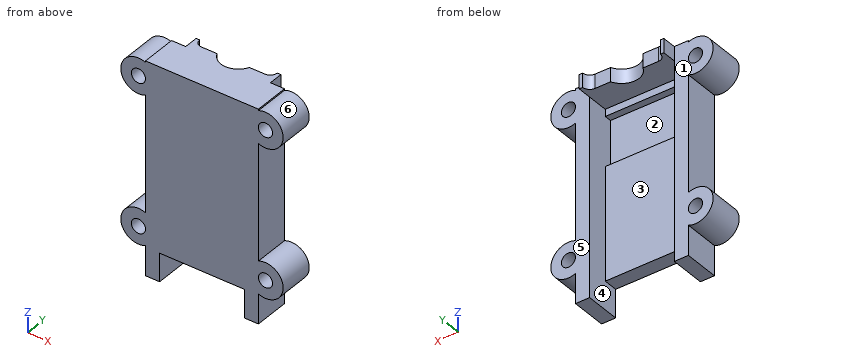
Autodesk Inventor part; units mm, degrees
ref_plane "YZ Plane" through (0, 0, 0) normal (1, 0, 0) x (0, 1, 0)
ref_plane "XZ Plane" through (0, 0, 0) normal (0, 1, 0) x (-1, 0, 0)
ref_plane "XY Plane" through (0, 0, 0) normal (0, 0, 1) x (1, 0, 0)
sketch "Sketch1" plane through (0, 0, 0) normal (0, 1, 0) x (-1, 0, 0)
  line L0 (8, 15) -> (-8, 15)
  line L1 (-8, 15) -> (-8, -15)
  line L2 (-8, -15) -> (8, -15)
  line L3 (8, -15) -> (8, 15)
  line L4 (8, 15) -> (-8, -15) construction
  line L5 (-8, 15) -> (8, -15) construction
  point P0 (0, 0)
  dimension "d0" = 16
  dimension "d1" = 30
extrude "Extrusion1" add sketch "Sketch1" along normal blind 2
sketch "Sketch2" plane through (0, 2, 0) normal (0, 1, 0) x (1, 0, 0)
  line L0 (8, 15) -> (-8, 15)
  line L1 (-6, 15) -> (6, 15)
  line L2 (6, 15) -> (6, -13)
  line L3 (6, -13) -> (-6, -13)
  line L4 (-6, -13) -> (-6, 15)
  line L5 (8, -15) -> (8, 15)
  line L6 (-8, 15) -> (-8, -15)
  line L7 (-8, -15) -> (8, -15)
  point P0 (0, 0)
  dimension "d4" = 2
  dimension "d5" = 2
  dimension "d6" = 2
extrude "Extrusion2" add sketch "Sketch2" along normal blind 3 contours L5 L7 L6 L0 L4 L3 L2
sketch "Sketch4" plane through (0, 5, 0) normal (0, 1, 0) x (1, 0, 0)
  line L0 (6, -13) -> (-6, -13)
  line L1 (-8, -15) -> (8, -15)
  line L2 (-6, -13) -> (6, -13)
  line L3 (6, -13) -> (6, -15)
  line L4 (6, -15) -> (-6, -15)
  line L5 (-6, -15) -> (-6, -13)
  line L6 (6, 15) -> (6, -13)
  point P0 (0, 0)
extrude "Extrusion3" add sketch "Sketch4" along normal blind 2
sketch "Sketch3" plane through (-8, 0, 15) normal (0, 0, 1) x (1, 0, 0)
  line L0 (14, 2) -> (2, 2) construction
  line L1 (2, 2) -> (14, 2) construction
  circle A0 centre (8, 7) radius 2.5
  line L2 (8, 11.4) -> (8, -1.9) construction
  line L3 (3.5, 7) -> (12.5, 7) construction
  circle A1 centre (3.5, 7) radius 1
  circle A2 centre (12.5, 7) radius 1
  line L4 (3.5, 8) -> (5.7087, 8)
  line L5 (12.5, 8) -> (10.2913, 8)
  line L6 (12.5, 6) -> (10.2913, 6)
  line L7 (5.7087, 6) -> (3.5, 6)
  point P0 (8, 0)
  dimension "d9" = 5
  dimension "d10" = 5
  dimension "d11" = 9
  dimension "d12" = 2
  dimension "d13" = 2
extrude "Extrusion4" cut sketch "Sketch3" against normal up to next
sketch "Sketch8" plane through (0, 2, 0) normal (0, 1, 0) x (1, 0, 0)
  line L0 (-6, 15) -> (-6, -13)
  line L1 (6, -13) -> (6, 15)
  line L2 (-6, 15) -> (6, 15)
  line L3 (6, 15) -> (6, 11)
  line L4 (6, 11) -> (-6, 11)
  line L5 (-6, 11) -> (-6, 15)
  line L6 (-2.2913, -13) -> (2.2913, -13)
  point P0 (0, 0)
  dimension "d28" = 24
extrude "Extrusion7" cut sketch "Sketch8" against normal up to next
sketch "Sketch9" plane through (0, 2, 0) normal (0, 1, 0) x (1, 0, 0)
  line L0 (-6, 11) -> (-6, -13)
  line L1 (6, -13) -> (6, 11)
  line L2 (-6, -12) -> (6, -12)
  line L3 (6, -12) -> (6, -5)
  line L4 (6, -5) -> (-6, -5)
  line L5 (-6, -5) -> (-6, -12)
  line L6 (-2.2913, -13) -> (2.2913, -13)
  point P0 (0, 0)
  point P1 (-6, -5)
  dimension "d31" = 1
  dimension "d32" = 7
extrude "Extrusion8" cut sketch "Sketch9" against normal blind 1
sketch "Sketch10" plane through (0, 0, 0) normal (0, -1, 0) x (1, 0, 0)
  circle A0 centre (-9, 12.5) radius 1
  circle A1 centre (-9, 12.5) radius 2.5
  line L0 (-8, -15) -> (-8, 15)
  line L1 (-8, 15) -> (8, 15)
  line L2 (8, 15) -> (8, -15)
  line L3 (-8, 15) -> (-6, 15)
  circle A2 centre (-9, -8.5) radius 1
  circle A3 centre (-9, -8.5) radius 2.5
  circle A4 centre (9, 12.5) radius 1
  circle A5 centre (9, 12.5) radius 2.5
  circle A6 centre (9, -8.5) radius 1
  circle A7 centre (9, -8.5) radius 2.5
  line L4 (6, -11) -> (-6, -11)
  point P0 (0, 0)
  point P1 (-8, -6)
  point P2 (10, 15)
  point P3 (10, -6)
  point P4 (-8, 12.5)
  point P5 (-8, 14.7913)
  point P6 (-8, 10.2087)
  point P7 (-8, -6.2087)
  point P8 (-8, -10.7913)
  point P9 (-8, -8.5)
  point P10 (8, 14.7913)
  point P11 (8, 12.5)
  point P12 (8, 10.2087)
  dimension "d35" = 2
  dimension "d36" = 1.5
  dimension "d38" = 16
  dimension "d41" = 21
  dimension "d44" = 18
  dimension "d49" = 26
extrude "Extrusion9" add sketch "Sketch10" against normal up to surface (5 mm away) contours L0 A1 | A7 L2 | L2 A7 | A5 L2 | L0 A3 picked at (-10.9649, 12.2158) picked at (10.9649, 12.2158) picked at (-10.9649, -8.7842)
equation "\"d5\" = d4"
equation "\"d6\" = d4"
equation "\"d41\" = -2 * d36 + d49 - d35"
properties part number "motor_top"
The model under review builds one solid part; all positions refer to its coordinate system, in mm. Face numbers are marked on the shaded views. A direction names the side the tool comes from. Give positions to 0.01 mm unless a question says otherwise; leave off trailing zeros. Write each loop counter-clockwise with the first axis right and the second up, starting at its lowest first coordinate (ties: lowest second). Pieces come first, ordered by that corner, then holes.
(1) Consider section D-D, the plane z = 12.5. Give the boundary of the cut face in (x, y), and give its area (3 significant figures).
(2) Tool access review of the marked faces 1, 2 and 3: name each direction out of +Z, -Z, +X, -X, +Y, -Y from which nothing blocks a thin tool from reaching the whole face with its end or side.
(3) To check wall thickness, follow L1, parallel to Z at x = -9, y = 2.6; L2, parallel to Z at x = 8.25, y = 0.5; L3, parallel to X at y = 3.5, z = -8. State the ranges of each line that lie inside material, in increasing order.
(4) The part is to be moulded in two halves that separate along X. For the marked faces 4, 5 and 6, say which applies: released by +X, released by -X, zero draft, split by the parting line, or undercut.
(5) For P1, Ø0.6, axis at x = 3.5, z = 14, coming from the +Y side; P2, Ø1, axis at x = 1, y = 1, coming from the -Z side; P3, Ø1.5, axis at x = 3.5, z = -3, coming from the +Y side; P4, Ø1.6, axis at x = 10, z = 6, coming from the +Y side, all flat-tipped, find the tip position at first contact; note any pin that passes through.
(6) Consider section A-A, the plane x = -9. Give the boundary of the cut face in (y, z).
(7) Consider section B-B, the plane z = 9.25. Give the boundary of the cut face in (x, y).
(8) Consider section C-C, the plane y = 3.75. Give the boundary of the cut face in (x, z).
Returned:
1. outline: (-11.5, 0) - (-10, 0) - (-10, 5) - (-11.5, 5) - close; (-8, 0) - (8, 0) - (8, 5) - (6, 5) - (6, 2) - (-6, 2) - (-6, 5) - (-8, 5) - close; (10, 0) - (11.5, 0) - (11.5, 5) - (10, 5) - close
1. area: 59.0 mm2
2. face 1: +Z, -Z, -X, +Y
2. face 2: +Y
2. face 3: -Z, +Y
3. L1: z = -11 to -9.5, -7.5 to -6, 10 to 11.5, 13.5 to 15
3. L2: z = -10.88 to -9.16, -7.84 to -6.12, 10.12 to 11.84, 13.16 to 14.88
3. L3: x = -11.45 to -9.87, -8.13 to -6, 6 to 8.13, 9.87 to 11.45
4. face 4: undercut
4. face 5: zero draft
4. face 6: undercut
5. P1: stops at y = 6
5. P2: stops at z = -11
5. P3: stops at y = 2
5. P4: passes through
6. outline: (0, -11) - (5, -11) - (5, -9.5) - (0, -9.5) - close; (0, -7.5) - (5, -7.5) - (5, -6) - (0, -6) - close; (0, 10) - (5, 10) - (5, 11.5) - (0, 11.5) - close; (0, 13.5) - (5, 13.5) - (5, 15) - (0, 15) - close
7. outline: (-8, 0) - (8, 0) - (8, 5) - (6, 5) - (6, 1) - (-6, 1) - (-6, 5) - (-8, 5) - close
8. outline: (-8, -15) - (-6, -15) - (-6, 13) - (6, 13) - (6, -15) - (8, -15) - (8, -10.79) arc R2.5 ccw (long way) to (8, -6.21) - (8, 10.21) arc R2.5 ccw (long way) to (8, 14.79) - (8, 15) - (-8, 15) - (-8, 14.79) arc R2.5 ccw (long way) to (-8, 10.21) - (-8, -6.21) arc R2.5 ccw (long way) to (-8, -10.79) - close; hole circle Ø2 at (-9, -8.5); hole circle Ø2 at (-9, 12.5); hole circle Ø2 at (9, -8.5); hole circle Ø2 at (9, 12.5)
